Geometry: final body of the model. Coordinates: model frame, mm. A direction names the side the tool comes from. Round coordinates to 2 decimals unless told otherwise and drop trailing zeros. Loops run counter-clockwise (first coordinate to the right, second up) from the corner with the lowest first, then second, coordinate; pieces in that order, holes last. Notation, with made-up numbers: (-10, 42.25) -> (49, 42.25) arc R18 ccw to (49, 77.25) -> close; hole circle Ø9 at (-28, 31). An arc over 180 degrees is marked (long way). Answer in a Markdown table with one row per item.
```python
from build123d import *

# Parameters (mm, degrees)
F0_R     = 20
F1_DEPTH = 15
F2_R     = 17.5
F2_R_2   = 2.5
F3_DEPTH = 6
F4_R     = 1.5
F5_DEPTH = 25
F6_R     = 17.5
F6_R_2   = 2.5
F7_DEPTH = 6


with BuildPart() as f1:
    # F0 (on Right) → F1 (new body)
    with BuildSketch(Plane.YZ):
        Circle(F0_R)
    extrude(amount=F1_DEPTH)

    # F2 (on face) → F3 (cut)
    with BuildSketch(Plane.YZ.offset(15)):
        Circle(F2_R)
        Circle(F2_R_2, mode=Mode.SUBTRACT)
    extrude(amount=-F3_DEPTH, mode=Mode.SUBTRACT)

    # F4 (on face) → F5 (cut)
    with BuildSketch(Plane.YZ.offset(15)):
        Circle(F4_R)
    extrude(amount=-F5_DEPTH, mode=Mode.SUBTRACT)

    # F6 (on face) → F7 (cut)
    with BuildSketch(Plane(origin=(0, 0, 0), x_dir=(0, -1, 0), z_dir=(-1, 0, 0))):
        Circle(F6_R)
        Circle(F6_R_2, mode=Mode.SUBTRACT)
    extrude(amount=-F7_DEPTH, mode=Mode.SUBTRACT)


solid = f1.part
```
Item 1: Cut plane D-D (y = 11.5). Output: boundary loops of the cut face in (x, z), then the cut area to 3 significant figures.
Answer:
| item | result |
|---|---|
| outline | (0, -16.36) -> (15, -16.36) -> (15, -13.19) -> (9, -13.19) -> (9, 13.19) -> (15, 13.19) -> (15, 16.36) -> (0, 16.36) -> (0, 13.19) -> (6, 13.19) -> (6, -13.19) -> (0, -13.19) -> close |
| area | 174 mm² |
Item 2: Draft query along Z for faces 1 (the face through (15, 0, -18)), 2 (the face through (7.395, -4.336, -19.524)), 3 (the face through (12.04, -0.54, -2.44)). Return one class per face: pulls with the +Z half, pulls with the -Z half, needs draft (parallel to the pull), parting line crosses it, or undercut.
Answer:
| item | result |
|---|---|
| face 1 | needs draft |
| face 2 | parting line crosses it |
| face 3 | undercut |
Item 3: Pin query (flat end, axial travel): pin 1 Ø5 at (x, z) = (4.5, 8) entering from -Y; pin 2 Ø1.5 at (x, y) = (1.5, -5.5) entering from +Z; pin 3 Ø8 at (x, z) = (7, 6) entering from -Y; pin 4 Ø5 at (x, z) = (4.5, -2) entering from +Y. Return the tip coordinate at first contact, or that it passes through.
Answer:
| item | result |
|---|---|
| pin 1 | stops at y = -19.23 |
| pin 2 | stops at z = 19.43 |
| pin 3 | stops at y = -19.9 |
| pin 4 | stops at y = 20 |
Item 4: Line query: probe 1 along Z at (x, y) = (11.5, 0); probe 2 along Y at (x, z) = (1.75, 2); probe 3 along Z at (x, y) = (7.5, 0). Output: solid intervals per line, ascending. Write a range as [from, to].
Answer:
| item | result |
|---|---|
| probe 1 | z = [-20, -17.5], [-2.5, -1.5], [1.5, 2.5], [17.5, 20] |
| probe 2 | y = [-19.9, -17.39], [-1.5, 1.5], [17.39, 19.9] |
| probe 3 | z = [-20, -1.5], [1.5, 20] |
Item 5: Cut plane A-A (z = 0). Output: boundary loops of the cut face in (x, y).
Answer:
| item | result |
|---|---|
| outline | (0, -20) -> (15, -20) -> (15, -17.5) -> (9, -17.5) -> (9, -2.5) -> (15, -2.5) -> (15, -1.5) -> (0, -1.5) -> (0, -2.5) -> (6, -2.5) -> (6, -17.5) -> (0, -17.5) -> close; (0, 1.5) -> (15, 1.5) -> (15, 2.5) -> (9, 2.5) -> (9, 17.5) -> (15, 17.5) -> (15, 20) -> (0, 20) -> (0, 17.5) -> (6, 17.5) -> (6, 2.5) -> (0, 2.5) -> close |
Item 6: Cut plane C-C (x = 4.25). Output: boundary loops of the cut face in (y, z), then the cut area to 3 significant figures.
Answer:
| item | result |
|---|---|
| outline | circle Ø40 at (0, 0); circle Ø5 at (0, 0); hole circle Ø35 at (0, 0); hole circle Ø3 at (0, 0) |
| area | 307 mm² |
Item 7: Reachability of faces 4 (the face through (0, 0, -2)), 5 (the face through (2.958, 13.887, -10.648)), 6 (the face through (9, 0, -4)) from +Z, -Z, +X, -X, +Y, -Y: full face, straight path, thin tool, end or side. Return the list, or none.
Answer:
| item | result |
|---|---|
| face 4 | +Z, -Z, -X, +Y, -Y |
| face 5 | -X |
| face 6 | +X |
